```python
from build123d import *

# Parameters (mm, degrees)
ESQUISSE1_W             = 12
ESQUISSE1_H             = 12
BOSS_EXTRU_1_DEPTH      = 50
ENL_V_MAT_EXTRU_1_DEPTH = 50
ESQUISSE3_R             = 1
ENL_V_MAT_EXTRU_2_DEPTH = 50


with BuildPart() as part:
    # Esquisse1 → Boss.-Extru.1 (new body)
    with BuildSketch(Plane(origin=(0, 0, 0), x_dir=(1, 0, 0), z_dir=(0, 1, 0))):
        Rectangle(ESQUISSE1_W, ESQUISSE1_H)
    extrude(amount=BOSS_EXTRU_1_DEPTH)

    # Esquisse2 → Enlèv. mat.-Extru.1 (cut)
    with BuildSketch(Plane(origin=(0, 50, 0), x_dir=(1, 0, 0), z_dir=(0, 1, 0))):
        Polygon((-5, -0.45), (-5, -1.45), (-4, -1.45), (-4, 1.45), (-5, 1.45), (-5, 0.45), (-6, 0.45), (-6, -0.45), align=None)
        Polygon((1.45, 5), (1.45, 4), (-1.45, 4), (-1.45, 5), (-0.45, 5), (-0.45, 6), (0.45, 6), (0.45, 5), align=None)
        Polygon((5, -1.45), (4, -1.45), (4, 1.45), (5, 1.45), (5, 0.45), (6, 0.45), (6, -0.45), (5, -0.45), align=None)
        Polygon((-1.45, -5), (-1.45, -4), (1.45, -4), (1.45, -5), (0.45, -5), (0.45, -6), (-0.45, -6), (-0.45, -5), align=None)
    extrude(amount=-ENL_V_MAT_EXTRU_1_DEPTH, mode=Mode.SUBTRACT)

    # Esquisse3 → Enlèv. mat.-Extru.2 (cut)
    with BuildSketch(Plane(origin=(0, 50, 0), x_dir=(1, 0, 0), z_dir=(0, 1, 0))):
        with Locations(Location((0, 0, 0), (0, 0, 270))):
            Circle(ESQUISSE3_R)
    extrude(amount=-ENL_V_MAT_EXTRU_2_DEPTH, mode=Mode.SUBTRACT)


solid = part.part
```
Geometry check sheet. Reference: the model listing, model coordinates, mm. A direction names the side the tool comes from. Give positions to 0.01 mm unless a question says otherwise; leave off trailing zeros. Write each loop counter-clockwise with the first axis right and the second up, starting at its lowest first coordinate (ties: lowest second). Pieces come first, ordered by that corner, then holes.
1) Access from +Z, -Z, +X, -X, +Y, -Y to the whole of each face (thin tool, end or side, straight path). Record for faces 4 (the flat face through (0.45, 25.4, -5.5)), 5 (the flat face through (5.5, 25.4, -0.45)), 6 (the flat face through (-5, 25, 1)), 7 (the flat face through (-0.45, 25.4, 5.5)).
2) Section check A-A, the plane z = 0. Record the boundary of the cut face in (x, y).
3) Material ranges on L1, parallel to Z at x = 5.75, y = 16.5; L2, parallel to X at y = 21.5, z = -0.75; L3, parallel to X at y = 21.5, z = -4.75, recorded low to high.
4) Release check for a two-part mould opening along X. For faces 1 (the flat face through (-1, 25, -5)), 2 (the flat face through (-6, 25, -3)), 3 (the flat face through (6, 25, 3)) record: pulls with the +X half, pulls with the -X half, needs draft (parallel to the pull), parting line crosses it, or undercut.
Computed:
1. face 4: -Z, +Y, -Y
1. face 5: +X, +Y, -Y
1. face 6: +Y, -Y
1. face 7: +Z, +Y, -Y
2. outline: (-4, 0) - (-1, 0) - (-1, 50) - (-4, 50) - close; (1, 0) - (4, 0) - (4, 50) - (1, 50) - close
3. L1: z = -6 to -0.45, 0.45 to 6
3. L2: x = -6 to -5, -4 to -0.66, 0.66 to 4, 5 to 6
3. L3: x = -6 to -1.45, 1.45 to 6
4. face 1: undercut
4. face 2: pulls with the -X half
4. face 3: pulls with the +X half
